from build123d import *

# Parameters (mm, degrees)
EXTRUDE_1_DEPTH      = 3
SKETCH_2_R           = 1.5
CUT_EXTRUDE_1_DEPTH  = 3
SKETCH_3_R           = 15
SKETCH_3_R_2         = 1.5
CUT_EXTRUDE_2_DEPTH  = 10
SKETCH_4_W           = 90
SKETCH_4_H           = 80
CUT_EXTRUDE_3_DEPTH  = 3
FILLET_3_R           = 6
CHAMFER_1_SIZE       = 8
SKETCH_7_R           = 1.5
CUT_EXTRUDE_6_DEPTH  = 10
CHAMFER_2_SIZE       = 20
SKETCH_8_R           = 1.5
CUT_EXTRUDE_7_DEPTH  = 10
SKETCH_9_R           = 1.5
CUT_EXTRUDE_8_DEPTH  = 10
SKETCH_10_R          = 1.5
CUT_EXTRUDE_9_DEPTH  = 10
CUT_EXTRUDE_10_DEPTH = 10


with BuildPart() as part:
    # 草图1 → 凸台-拉伸1 (new body)
    with BuildSketch(Plane(origin=(0, 0, 0), x_dir=(1, 0, 0), z_dir=(0, 1, 0))):
        Polygon((-50, -51), (-50, -105), (50, -105), (50, -51), (145, -51), (145, 51), (50, 51), (50, 105), (-50, 105), (-50, 51), (-145, 51), (-145, -51), align=None)
    extrude(amount=EXTRUDE_1_DEPTH)

    # 草图2 → 切除-拉伸1 (cut)
    with BuildSketch(Plane(origin=(0, 3, 0), x_dir=(1, 0, 0), z_dir=(0, 1, 0))):
        with Locations(Location((111, 42, 0), (0, 0, 270))):
            Circle(SKETCH_2_R)
        with Locations(Location((81, 42, 0), (0, 0, 270))):
            Circle(SKETCH_2_R)
        with Locations(Location((81, 18, 0), (0, 0, 270))):
            Circle(SKETCH_2_R)
        with Locations(Location((111, 18, 0), (0, 0, 270))):
            Circle(SKETCH_2_R)
        with Locations(Location((111, -18, 0), (0, 0, 90))):
            Circle(SKETCH_2_R)
        with Locations(Location((111, -42, 0), (0, 0, 90))):
            Circle(SKETCH_2_R)
        with Locations(Location((81, -18, 0), (0, 0, 90))):
            Circle(SKETCH_2_R)
        with Locations(Location((81, -42, 0), (0, 0, 90))):
            Circle(SKETCH_2_R)
        with Locations(Location((-81, -42, 0), (0, 0, 270))):
            Circle(SKETCH_2_R)
        with Locations(Location((-81, -18, 0), (0, 0, 270))):
            Circle(SKETCH_2_R)
        with Locations(Location((-111, -42, 0), (0, 0, 270))):
            Circle(SKETCH_2_R)
        with Locations(Location((-111, -18, 0), (0, 0, 270))):
            Circle(SKETCH_2_R)
        with Locations(Location((-111, 18, 0), (0, 0, 90))):
            Circle(SKETCH_2_R)
        with Locations(Location((-81, 18, 0), (0, 0, 90))):
            Circle(SKETCH_2_R)
        with Locations(Location((-81, 42, 0), (0, 0, 90))):
            Circle(SKETCH_2_R)
        with Locations(Location((-111, 42, 0), (0, 0, 90))):
            Circle(SKETCH_2_R)
    extrude(amount=-CUT_EXTRUDE_1_DEPTH, mode=Mode.SUBTRACT)

    # 草图3 → 切除-拉伸2 (cut)
    with BuildSketch(Plane(origin=(0, 3, 0), x_dir=(1, 0, 0), z_dir=(0, 1, 0))):
        with Locations(Location((0, 77, 0), (0, 0, 270))):
            Circle(SKETCH_3_R)
        with Locations(Location((15.11, 97, 0), (0, 0, 270))):
            Circle(SKETCH_3_R_2)
        with Locations(Location((15.11, 57, 0), (0, 0, 270))):
            Circle(SKETCH_3_R_2)
        with Locations(Location((-34.89, 57, 0), (0, 0, 270))):
            Circle(SKETCH_3_R_2)
        with Locations(Location((-34.89, 97, 0), (0, 0, 270))):
            Circle(SKETCH_3_R_2)
        with Locations(Location((-27, -70.5, 0), (0, 0, 270))):
            Circle(SKETCH_3_R_2)
        with Locations(Location((32, -67, 0), (0, 0, 270))):
            Circle(SKETCH_3_R_2)
        with Locations(Location((-27, -100.5, 0), (0, 0, 270))):
            Circle(SKETCH_3_R_2)
        with Locations(Location((33, -100.5, 0), (0, 0, 270))):
            Circle(SKETCH_3_R_2)
    extrude(amount=-CUT_EXTRUDE_2_DEPTH, mode=Mode.SUBTRACT)

    # 草图4 → 切除-拉伸3 (cut)
    with BuildSketch(Plane(origin=(0, 3, 0), x_dir=(1, 0, 0), z_dir=(0, 1, 0))):
        Rectangle(SKETCH_4_W, SKETCH_4_H)
    extrude(amount=-CUT_EXTRUDE_3_DEPTH, mode=Mode.SUBTRACT)

    # 圆角3
    fillet_3_edges = [part.edges().sort_by_distance(p)[0] for p in [
        (-145, 1.5, 51),
        (-145, 1.5, -51),
        (-50, 1.5, -105),
        (50, 1.5, -105),
        (145, 1.5, -51),
        (145, 1.5, 51),
        (50, 1.5, 105),
        (-50, 1.5, 105),
    ]]
    fillet(fillet_3_edges, radius=FILLET_3_R)

    # 倒角1
    chamfer_1_edges = [part.edges().sort_by_distance(p)[0] for p in [
        (-50, 1.5, 51),
        (-50, 1.5, -51),
        (50, 1.5, -51),
        (50, 1.5, 51),
    ]]
    chamfer(chamfer_1_edges, length=CHAMFER_1_SIZE)

    # 草图7 → 切除-拉伸6 (cut)
    with BuildSketch(Plane(origin=(0, 3, 0), x_dir=(1, 0, 0), z_dir=(0, 1, 0))):
        with Locations(Location((47, 27.5, 0), (0, 0, 270))):
            Circle(SKETCH_7_R)
        with Locations(Location((47, -27.5, 0), (0, 0, 270))):
            Circle(SKETCH_7_R)
        with Locations(Location((69, 27.5, 0), (0, 0, 270))):
            Circle(SKETCH_7_R)
        with Locations(Location((69, -27.5, 0), (0, 0, 270))):
            Circle(SKETCH_7_R)
        with BuildLine():
            Line((-65, -20), (-65, 20))
            ThreePointArc((-65, 20), (-60, 25), (-55, 20))
            Line((-55, 20), (-55, -20))
            ThreePointArc((-55, -20), (-60, -25), (-65, -20))
        make_face()
        with BuildLine():
            Line((65, -20), (65, 20))
            ThreePointArc((65, 20), (60, 25), (55, 20))
            Line((55, 20), (55, -20))
            ThreePointArc((55, -20), (60, -25), (65, -20))
        make_face()
        with BuildLine():
            Line((-141, -15), (-141, 15))
            ThreePointArc((-141, 15), (-137, 19), (-133, 15))
            Line((-133, 15), (-133, -15))
            ThreePointArc((-133, -15), (-137, -19), (-141, -15))
        make_face()
        with BuildLine():
            Line((129, 27), (129, 41))
            ThreePointArc((129, 41), (134, 46), (139, 41))
            Line((139, 41), (139, 27))
            ThreePointArc((139, 27), (134, 22), (129, 27))
        make_face()
        with BuildLine():
            Line((129, -27), (129, -41))
            ThreePointArc((129, -41), (134, -46), (139, -41))
            Line((139, -41), (139, -27))
            ThreePointArc((139, -27), (134, -22), (129, -27))
        make_face()
    extrude(amount=-CUT_EXTRUDE_6_DEPTH, mode=Mode.SUBTRACT)

    # 倒角2
    chamfer_2_edges = [part.edges().sort_by_distance(p)[0] for p in [
        (45, 1.5, -40),
        (45, 1.5, 40),
        (-45, 1.5, 40),
        (-45, 1.5, -40),
    ]]
    chamfer(chamfer_2_edges, length=CHAMFER_2_SIZE)

    # 草图8 → 切除-拉伸7 (cut)
    with BuildSketch(Plane(origin=(0, 3, 0), x_dir=(1, 0, 0), z_dir=(0, 1, 0))):
        with Locations(Location((-127.5, 23, 0), (0, 0, 270))):
            Circle(SKETCH_8_R)
        with Locations(Location((-127.5, -35, 0), (0, 0, 270))):
            Circle(SKETCH_8_R)
        with Locations(Location((-141, 30, 0), (0, 0, 270))):
            Circle(SKETCH_8_R)
        with Locations(Location((-133, 30, 0), (0, 0, 270))):
            Circle(SKETCH_8_R)
    extrude(amount=-CUT_EXTRUDE_7_DEPTH, mode=Mode.SUBTRACT)

    # 草图9 → 切除-拉伸8 (cut)
    with BuildSketch(Plane(origin=(0, 3, 0), x_dir=(1, 0, 0), z_dir=(0, 1, 0))):
        with Locations(Location((43.343145751, 44, 0), (0, 0, 270))):
            Circle(SKETCH_9_R)
        with Locations(Location((49, 38.343145751, 0), (0, 0, 270))):
            Circle(SKETCH_9_R)
        with Locations(Location((49, -38.343145751, 0), (0, 0, 270))):
            Circle(SKETCH_9_R)
        with Locations(Location((43.343145751, -44, 0), (0, 0, 270))):
            Circle(SKETCH_9_R)
        with Locations(Location((-43.343145751, -44, 0), (0, 0, 270))):
            Circle(SKETCH_9_R)
        with Locations(Location((-49, -38.343145751, 0), (0, 0, 270))):
            Circle(SKETCH_9_R)
        with Locations(Location((-49, 38.343145751, 0), (0, 0, 270))):
            Circle(SKETCH_9_R)
        with Locations(Location((-43.343145751, 44, 0), (0, 0, 270))):
            Circle(SKETCH_9_R)
        with Locations(Location((-38, -95, 0), (0, 0, 270))):
            Circle(SKETCH_9_R)
        with Locations(Location((38, -95, 0), (0, 0, 270))):
            Circle(SKETCH_9_R)
        with Locations(Location((-62, 40, 0), (0, 0, 270))):
            Circle(SKETCH_9_R)
        with Locations(Location((-62, -40, 0), (0, 0, 270))):
            Circle(SKETCH_9_R)
    extrude(amount=-CUT_EXTRUDE_8_DEPTH, mode=Mode.SUBTRACT)

    # 草图10 → 切除-拉伸9 (cut)
    with BuildSketch(Plane(origin=(0, 3, 0), x_dir=(1, 0, 0), z_dir=(0, 1, 0))):
        with Locations(Location((76.1, 5, 0), (0, 0, 270))):
            Circle(SKETCH_10_R)
        with Locations(Location((133.1, 15, 0), (0, 0, 270))):
            Circle(SKETCH_10_R)
        with Locations(Location((133.1, -15, 0), (0, 0, 270))):
            Circle(SKETCH_10_R)
        with Locations(Location((76.1, -5, 0), (0, 0, 270))):
            Circle(SKETCH_10_R)
    extrude(amount=-CUT_EXTRUDE_9_DEPTH, mode=Mode.SUBTRACT)

    # 草图11 → 切除-拉伸10 (cut)
    with BuildSketch(Plane(origin=(0, 3, 0), x_dir=(1, 0, 0), z_dir=(0, 1, 0))):
        with BuildLine():
            Line((-21.514718626, -57.878679656), (-32.121320344, -68.485281374))
            ThreePointArc((-32.121320344, -68.485281374), (-38.485281374, -68.485281374), (-38.485281374, -62.121320344))
            Line((-38.485281374, -62.121320344), (-27.878679656, -51.514718626))
            ThreePointArc((-27.878679656, -51.514718626), (-21.514718626, -51.514718626), (-21.514718626, -57.878679656))
        make_face()
        with BuildLine():
            Line((14, -45), (26, -45))
            ThreePointArc((26, -45), (31, -50), (26, -55))
            Line((26, -55), (14, -55))
            ThreePointArc((14, -55), (9, -50), (14, -45))
        make_face()
        with BuildLine():
            Line((-15, -81), (15, -81))
            ThreePointArc((15, -81), (20, -86), (15, -91))
            Line((15, -91), (-15, -91))
            ThreePointArc((-15, -91), (-20, -86), (-15, -81))
        make_face()
    extrude(amount=-CUT_EXTRUDE_10_DEPTH, mode=Mode.SUBTRACT)


solid = part.part
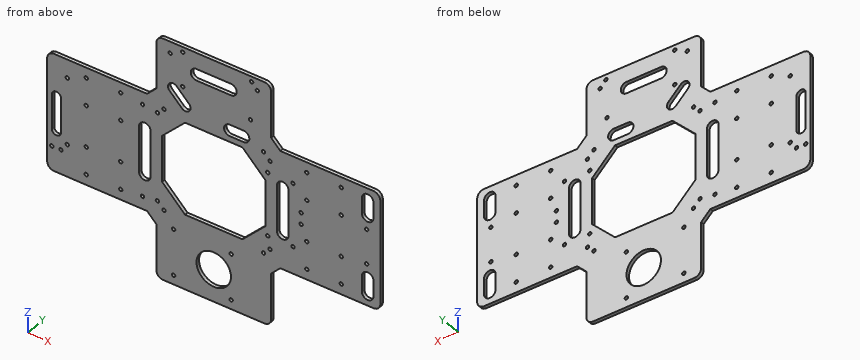
The listing builds one solid part. Answer for the finished solid, in the listing's coordinates (mm). Coordinates: 2 decimals unless noted, no trailing zeros. Write each loop counter-clockwise with the first axis right and the second up, starting at its lowest first coordinate (ties: lowest second). Pieces come first, ordered by that corner, then holes. Notation, with made-up numbers: M -7.75,-28 L 40.25,-28 A24 ccw 40.25,2 Z; hole C 57,38.25 d5. An arc over 180 degrees is marked long. Write each question's results on one line, items separated by ' | '.
Item 1: The part is cut by section D-D on z = -71. Determine the outline of the cut face in (x, y).
Answer below:
outline: M -50,0 L -13.75,0 L -13.75,3 L -50,3 Z; M 13.75,0 L 50,0 L 50,3 L 13.75,3 Z
Item 2: The part is cut by section C-C on y = 1.6. State how many separate pieces and enclosed holes the cut face has, and give its area (3 significant figures).
Answer below:
separate pieces: 1 | enclosed holes: 58 | area: 30,500 mm2
Item 3: Consider probe 1 along X at (y, z) = (0.95, -10); probe 2 along X at (y, z) = (1.75, -97); probe 3 along Z at (x, y) = (-111, 1.7). Determine where each line is inside the solid, lowest interval first. Write a range as [from, to].
Answer below:
probe 1: [-145, -141], [-133, -65], [-55, -45], [45, 55], [65, 145] | probe 2: [-50, -36.39], [-33.39, 13.61], [16.61, 50] | probe 3: [-51, -43.5], [-40.5, -19.5], [-16.5, 16.5], [19.5, 40.5], [43.5, 51]
Item 4: The part is cut by section A-A on z = 85. Determine the outline of the cut face in (x, y), and give its area (3 significant figures).
Answer below:
outline: M -50,0 L -19.9,0 L -19.9,3 L -50,3 Z; M 19.9,0 L 50,0 L 50,3 L 19.9,3 Z | area: 181 mm2
Item 5: The part is cut by section B-B on x = -11. Determine the outline of the cut face in (y, z), and give its area (3 significant figures).
Answer below:
outline: M 0,-105 L 3,-105 L 3,-87.2 L 0,-87.2 Z; M 0,-66.8 L 3,-66.8 L 3,-40 L 0,-40 Z; M 0,40 L 3,40 L 3,81 L 0,81 Z; M 0,91 L 3,91 L 3,105 L 0,105 Z | area: 299 mm2
Item 6: Given P1, Ø1.5, axis at x = -84.5, y = 2, coming from the -Z side; P2, Ø0.9, axis at y = 2, z = 77.5, coming from the -X side; P3, Ø3.5, axis at x = 15.11, z = -97, coming from the +Y side, each flat-ended and moving along its own axis, determine where each tip first touches the part or whether it passes through.
Answer below:
P1: z = -51 | P2: x = -50 | P3: y = 3
